Geometry: final body of the model. Coordinates: model frame, mm. Face numbers are marked on the shaded views. A direction names the side the tool comes from. Coordinates: 2 decimals unless noted, no trailing zeros. Write each loop counter-clockwise with the first axis right and the second up, starting at its lowest first coordinate (ties: lowest second). Pieces come first, ordered by that corner, then holes.
from build123d import *

# Parameters (mm, degrees)
F1_DEPTH      = 457.2
F1_DEPTH_BACK = 457.2


with BuildPart() as f1:
    # F0 (on Right) → F1 (new body, two sides)
    with BuildSketch(Plane.YZ) as f1_sk:
        with BuildLine():
            Line((101.6, 71.4375), (101.6, 76.2))
            Line((101.6, 76.2), (6.35, 76.2))
            ThreePointArc((6.35, 76.2), (1.8598719395, 74.3401280605), (0, 69.85))
            Line((0, 69.85), (0, 0))
            Line((0, 0), (0, -69.85))
            ThreePointArc((0, -69.85), (1.8598719395, -74.3401280605), (6.35, -76.2))
            Line((6.35, -76.2), (101.6, -76.2))
            Line((101.6, -76.2), (101.6, -71.4375))
            Line((101.6, -71.4375), (9.525, -71.4375))
            ThreePointArc((9.525, -71.4375), (6.1574039546, -70.0425960454), (4.7625, -66.675))
            Line((4.7625, -66.675), (4.7625, 0))
            Line((4.7625, 0), (4.7625, 66.675))
            ThreePointArc((4.7625, 66.675), (6.1574039546, 70.0425960454), (9.525, 71.4375))
            Line((9.525, 71.4375), (101.6, 71.4375))
        make_face()
    extrude(amount=-F1_DEPTH)
    extrude(f1_sk.sketch, amount=F1_DEPTH_BACK)


solid = f1.part
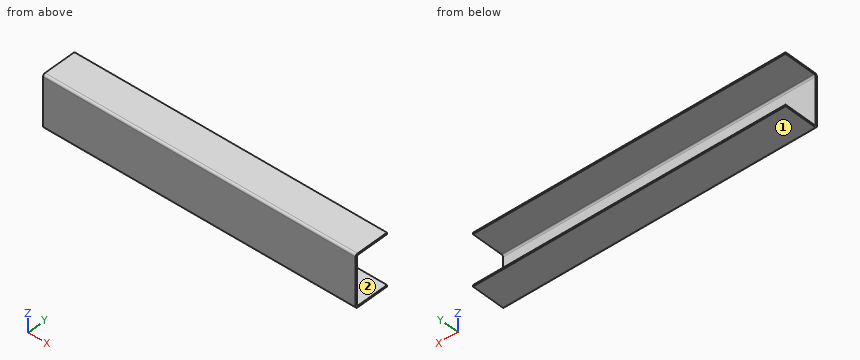
Item 1: Section A-A, the plane y = 62. Output: boundary loops of the cut face in (x, z), plus the area to 3 significant figures.
Derived:
outline: (-457.2, -76.2) - (457.2, -76.2) - (457.2, -71.44) - (-457.2, -71.44) - close; (-457.2, 71.44) - (457.2, 71.44) - (457.2, 76.2) - (-457.2, 76.2) - close
area: 8,710 mm2
Item 2: Pin query (flat end, axial travel): pin 1 (1.5 mm diameter, centred on x = -108.5, z = -40, fed in from +Y). Return the tip coordinate at first contact, or that it passes through.
Derived:
pin 1: stops at y = 4.76
Item 3: Material intervals for probe 1 along Z at (x, y) = (20, 79.5); probe 2 along Y at (x, z) = (359, 49); probe 3 along Z at (x, y) = (407.5, 6.5), sorted ascending.
Derived:
probe 1: z = -76.2 to -71.44, 71.44 to 76.2
probe 2: y = 0 to 4.76
probe 3: z = -76.2 to -70.35, 70.35 to 76.2
Item 4: Set-up query: the marked faces 1 and 2. Return all of +Z, -Z, +X, -X, +Y, -Y with unobstructed straight access to the full face (end or side cutting, diameter ignored); none if empty.
Derived:
face 1: -Z, +X, -X, +Y, -Y
face 2: +X, -X, +Y
Item 5: Section C-C, the plane z = 55.5. Output: boundary loops of the cut face in (x, y).
Derived:
outline: (-457.2, 0) - (457.2, 0) - (457.2, 4.76) - (-457.2, 4.76) - close
